Check sheet for the drawn part. Datum: minimum x, y, z corner. Units: mm. A direction names the side the tool comes from. Give positions to 0.01 mm unless a question says otherwise; leave off trailing zeros. Write each loop counter-clockwise with the first axis right and the second up, starting at its lowest first coordinate (ties: lowest second). Pieces come first, ordered by that corner, then holes. Notation, with made-up numbers: (-9, 84) - (10, 84) arc R35 cw to (10, 123) - close; hole circle Ø7 at (9, 71.25). An arc over 180 degrees is marked (long way). One line per question, with ' | ' between items. Start each with the question number.
Q1. Section check A-A on x = 78. Record the boundary of the cut face in (y, z).
Q2. Section check C-C on y = 17. Record the boundary of the cut face in (x, z).
Q3. Gauge pin test, flat ends, axial feed: P1, Ø2, axis at y = 19.5, z = 5.5, coming from the -X side; P2, Ø1, axis at y = 14, z = 8, coming from the -X side; P3, Ø3, axis at y = 4, z = 1.5, coming from the -X side. Record the tip position at first contact, or that the pin passes through.
Q4. Release check for a two-part mould opening along Y. For the marked faces 1, 2, 3 and 4 record: +Y half, -Y half, draft (parallel to the pull), parting line (faces both ways), or undercut.
Q5. Set-up check for the marked faces 5 and 6: record each of +Z, -Z, +X, -X, +Y, -Y from which the full face is reachable in a straight line by a thin tool's end or side.
Q6. Thickness scan on L1, parallel to Y at x = 145, z = 5; L2, parallel to X at y = 11.5, z = 9.5; L3, parallel to Y at x = 165, z = 1.75. Record the ranges inside material, lowest first. Write a range as [from, to].
Q7. Section check B-B on z = 3.75. Record the boundary of the cut face in (x, y), and give its area (3 significant figures).
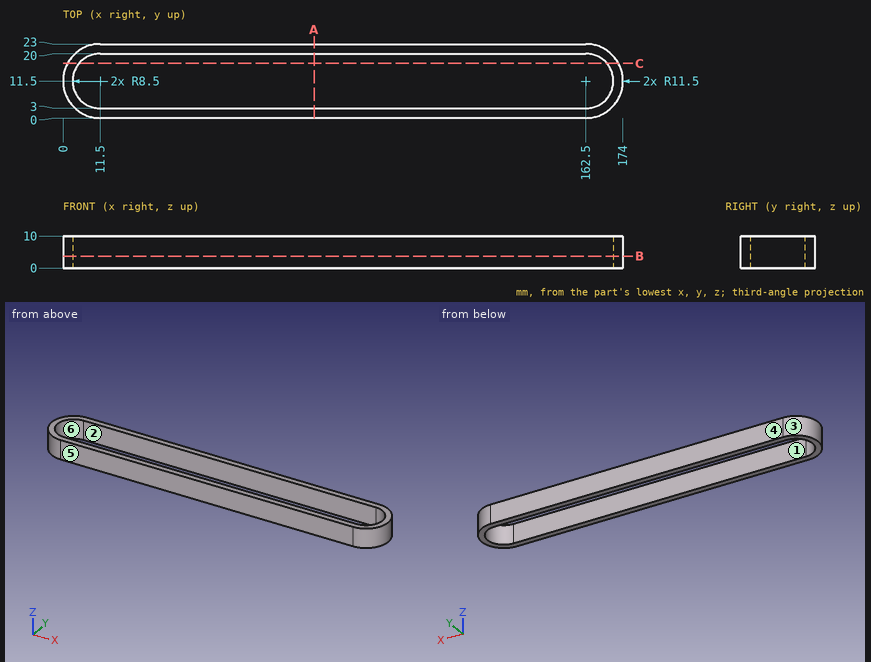
Working result:
1) outline: (0, 0) - (3, 0) - (3, 10) - (0, 10) - close; (20, 0) - (23, 0) - (23, 10) - (20, 10) - close
2) outline: (1.4, 0) - (5.02, 0) - (5.02, 10) - (1.4, 10) - close; (168.98, 0) - (172.6, 0) - (172.6, 10) - (168.98, 10) - close
3) P1: stops at x = 2.38 | P2: stops at x = 0.18 | P3: stops at x = 1.69
4) face 1: undercut | face 2: undercut | face 3: parting line | face 4: +Y half
5) face 5: +Z, -Z, +X, -X, -Y | face 6: +Z, -Z
6) L1: y = [0, 3], [20, 23] | L2: x = [0, 3], [171, 174] | L3: y = [0.28, 3.38], [19.62, 22.72]
7) outline: (11.5, 0) - (162.5, 0) arc R11.5 ccw to (162.5, 23) - (11.5, 23) arc R11.5 ccw to start; hole (11.5, 3) - (162.5, 3) arc R8.5 ccw to (162.5, 20) - (11.5, 20) arc R8.5 ccw to start | area: 1,090 mm2
